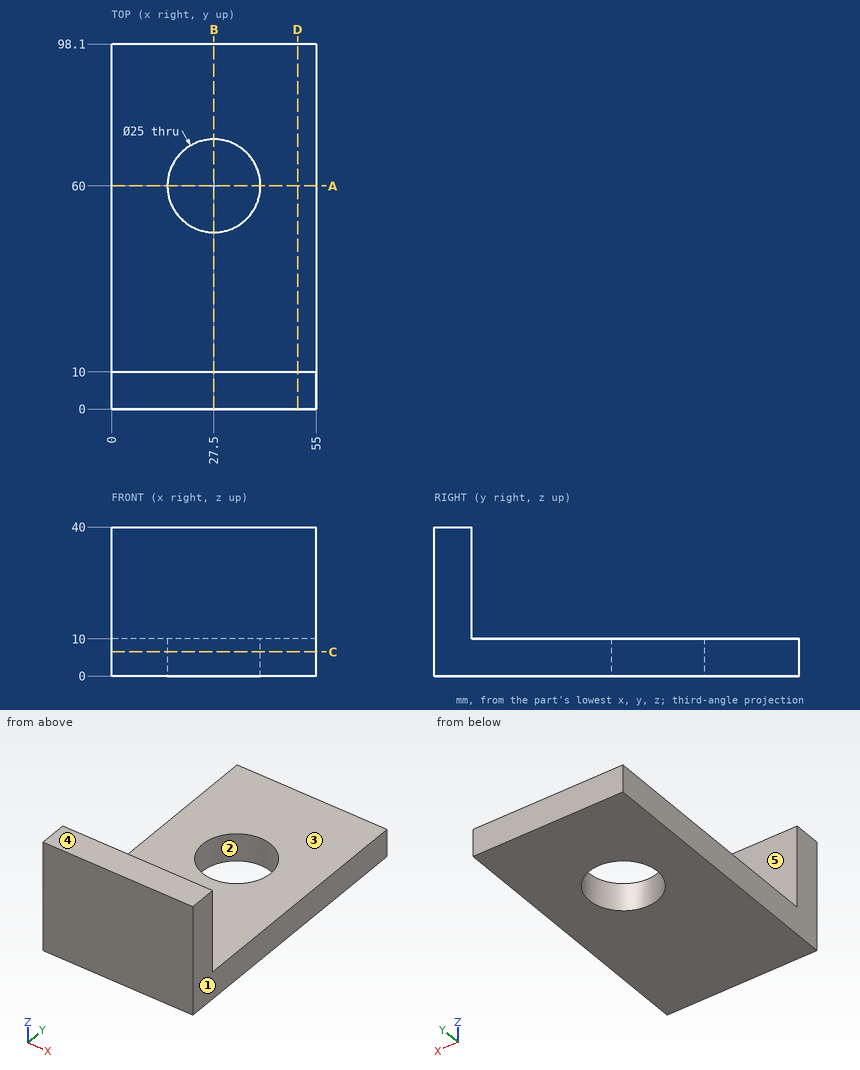
Can you work these out from the drawing? Everything is in mm from the part's minimum corner. A direction names the side the tool comes from. Coordinates: 2 decimals unless noted, no trailing zeros. Loops run counter-clockwise (first coordinate to the right, second up) from the corner with the lowest first, then second, coordinate; pieces in that order, holes last.
1) Imagine slicing it at C-C on z = 6.5. List the corners of the cut face in (x, y) for me.
2) Imagine slicing it at B-B on x = 27.5. List the corners of the cut face in (y, z) for me, plus the area to 3 significant figures.
3) Imagine slicing it at A-A on y = 60. List the corners of the cut face in (x, z) for me, plus the area to 3 significant figures.
4) Thinking about a two-plate mould opening in X: for the marked faces 1, 2 and 3, which applies, pulls with the +X half, pulls with the -X half, needs draft (parallel to the pull), parting line crosses it, or undercut?
5) Imagine slicing it at D-D on x = 50. List the corners of the cut face in (y, z) for me.
6) I need wall thicknesses on probe 1 along Y at (x, z) = (27.5, 7.5); probe 2 along Y at (x, z) = (27.5, 27). Which ranges of each line are inside material? Lowest first, please.
7) Which directions (+Z, -Z, +X, -X, +Y, -Y) give clear straight access to the entire face, cutting with the end or side of a thin tool? Please do the marked faces 4 and 5.
8) For pin 1 (10 mm diameter, centred on y = 87.5, z = 13, fed in from -X); pin 2 (3 mm diameter, centred on x = 6, z = 32.5, fed in from +Y); pin 3 (3 mm diameter, centred on x = 7.5, y = 81.5, fed in from +Z); pin 4 (22.5 mm diameter, centred on x = 27.5, y = 60, fed in from -Z), each with a flat end and sliding along its axis, tell me the tip position at first contact or that it passes through.
Completed:
1. outline: (0, 0) - (55, 0) - (55, 98.1) - (0, 98.1) - close; hole circle Ø25 at (27.5, 60)
2. outline: (0, 0) - (47.5, 0) - (47.5, 10) - (10, 10) - (10, 40) - (0, 40) - close; (72.5, 0) - (98.1, 0) - (98.1, 10) - (72.5, 10) - close
2. area: 1,030 mm2
3. outline: (0, 0) - (15, 0) - (15, 10) - (0, 10) - close; (40, 0) - (55, 0) - (55, 10) - (40, 10) - close
3. area: 300 mm2
4. face 1: pulls with the +X half
4. face 2: undercut
4. face 3: needs draft
5. outline: (0, 0) - (98.1, 0) - (98.1, 10) - (10, 10) - (10, 40) - (0, 40) - close
6. probe 1: y = 0 to 47.5, 72.5 to 98.1
6. probe 2: y = 0 to 10
7. face 4: +Z, +X, -X, +Y, -Y
7. face 5: +Z, +X, -X, +Y
8. pin 1: stops at x = 0
8. pin 2: stops at y = 10
8. pin 3: stops at z = 10
8. pin 4: passes through
